Design review of the part built by this model. Coordinates are the model's own, in mm. A direction names the side the tool comes from. Give positions to 0.01 mm unless a question says otherwise; leave off trailing zeros. Loops run counter-clockwise (first coordinate to the right, second up) from the corner with the lowest first, then second, coordinate; pieces in that order, holes last. Notation, with made-up numbers: (-14, 12) - (-1, 12) arc R16 cw to (-1, 35) - close; hole circle Ø2 at (42, -3.75). An arc over 180 degrees is marked (long way). Write each question's results on one line, items separated by ' | '.
```python
from build123d import *

# Parameters (mm, degrees)
DODANIE_WYCI_GNI_CIE1_DEPTH = 900
SKORUPA1_T                  = -10
SZKIC4_R                    = 12
DODANIE_WYCI_GNI_CIE3_DEPTH = 15
SZKIC6_R                    = 12
SZKIC6_R_2                  = 8.15
DODANIE_WYCI_GNI_CIE4_DEPTH = 10
ZAOKR_GLENIE3_R             = 45
SZKIC8_R                    = 20
WYTNIJ_WYCI_GNI_CIE1_DEPTH  = 7.5
SZKIC11_R                   = 20
WYTNIJ_WYCI_GNI_CIE2_DEPTH  = 5
SZKIC12_R                   = 20
WYTNIJ_WYCI_GNI_CIE3_DEPTH  = 5
SZKIC13_R                   = 20
WYTNIJ_WYCI_GNI_CIE4_DEPTH  = 7.5
ZAOKR_GLENIE4_R             = 10
ZAOKR_GLENIE5_R             = 10


with BuildPart() as part:
    # Szkic1 → Dodanie-wyciągnięcie1 (new body)
    with BuildSketch(Plane.XY):
        with BuildLine():
            Line((-469.846310393, -171.010071663), (0, 0))
            Line((0, 0), (0, -500))
            ThreePointArc((0, -500), (-286.788218176, -409.576022144), (-469.846310393, -171.010071663))
        make_face()
    extrude(amount=DODANIE_WYCI_GNI_CIE1_DEPTH)

    # Skorupa1
    skorupa1_openings = [part.faces().sort_by_distance(p)[0] for p in [
        (-179.521279962, -256.382958146, 900),
        (-179.521279962, -256.382958146, 0),
        (-234.923155196, -85.505035831, 450),
        (0, -250, 450),
    ]]
    offset(amount=SKORUPA1_T, openings=skorupa1_openings, kind=Kind.INTERSECTION)

    # Szkic4 → Dodanie-wyciągnięcie3 (add)
    with BuildSketch(Plane(origin=(0, 0, 0), x_dir=(-1, 0, 0), z_dir=(0, 0, -1))):
        with BuildLine():
            Line((0, -20), (0, -490))
            ThreePointArc((0, -490), (281.052453812, -401.384501702), (460.449384185, -167.58987023))
            Line((460.449384185, -167.58987023), (18.793852416, -6.840402867))
            ThreePointArc((18.793852416, -6.840402867), (-11.471528727, 16.383040886), (0, -20))
        make_face()
        Circle(SZKIC4_R, mode=Mode.SUBTRACT)
    dodanie_wyci_gni_cie3 = extrude(amount=-DODANIE_WYCI_GNI_CIE3_DEPTH)

    # Lustro1: Dodanie-wyciągnięcie3 across plane
    add(dodanie_wyci_gni_cie3.mirror(Plane.XY.offset(450)))

    # Szkic6 → Dodanie-wyciągnięcie4 (add)
    with BuildSketch(Plane.XY.offset(440)):
        with BuildLine():
            Line((-18.793852416, -6.840402867), (-460.449384185, -167.58987023))
            ThreePointArc((-460.449384185, -167.58987023), (-281.052453812, -401.384501702), (0, -490))
            Line((0, -490), (0, -20))
            ThreePointArc((0, -20), (11.471528727, 16.383040886), (-18.793852416, -6.840402867))
        make_face()
        with Locations(Location((0, 0, 0), (0, 0, 180))):
            Circle(SZKIC6_R, mode=Mode.SUBTRACT)
        with Locations((-190.094997116, -90.472476083)):
            Circle(SZKIC6_R_2, mode=Mode.SUBTRACT)
        with BuildLine():
            Line((-20, -28.562960135), (-20, -469.574275275))
            ThreePointArc((-20, -469.574275275), (-269.580925085, -385.001460816), (-434.41507852, -179.397713347))
            Line((-434.41507852, -179.397713347), (-208.888849532, -97.312878949))
            ThreePointArc((-208.888849532, -97.312878949), (-183.254594249, -109.266328498), (-171.3011447, -83.632073216))
            Line((-171.3011447, -83.632073216), (-20, -28.562960135))
        make_face(mode=Mode.SUBTRACT)
    dodanie_wyci_gni_cie4 = extrude(amount=-DODANIE_WYCI_GNI_CIE4_DEPTH)

    # Lustro6: Dodanie-wyciągnięcie4 across plane
    add(dodanie_wyci_gni_cie4.mirror(Plane.XY.offset(450)))

    # Zaokrąglenie3
    zaokr_glenie3_edges = [part.edges().sort_by_distance(p)[0] for p in [
        (-434.41507852, -179.397713347, 435),
        (-20, -28.562960135, 435),
        (-20, -469.574275275, 435),
        (-20, -469.574275275, 465),
        (-20, -28.562960135, 465),
        (-434.41507852, -179.397713347, 465),
    ]]
    fillet(zaokr_glenie3_edges, radius=ZAOKR_GLENIE3_R)

    # Szkic8 → Wytnij-wyciągnięcie1 (cut)
    with BuildSketch(Plane(origin=(0, 0, 0), x_dir=(-1, 0, 0), z_dir=(0, 0, -1))):
        Circle(SZKIC8_R)
    extrude(amount=-WYTNIJ_WYCI_GNI_CIE1_DEPTH, mode=Mode.SUBTRACT)

    # Szkic11 → Wytnij-wyciągnięcie2 (cut)
    with BuildSketch(Plane(origin=(0, 0, 430), x_dir=(-1, 0, 0), z_dir=(0, 0, -1))):
        Circle(SZKIC11_R)
    extrude(amount=-WYTNIJ_WYCI_GNI_CIE2_DEPTH, mode=Mode.SUBTRACT)

    # Szkic12 → Wytnij-wyciągnięcie3 (cut)
    with BuildSketch(Plane(origin=(0, 0, 460), x_dir=(-1, 0, 0), z_dir=(0, 0, -1))):
        Circle(SZKIC12_R)
    extrude(amount=-WYTNIJ_WYCI_GNI_CIE3_DEPTH, mode=Mode.SUBTRACT)

    # Szkic13 → Wytnij-wyciągnięcie4 (cut)
    with BuildSketch(Plane(origin=(0, 0, 885), x_dir=(-1, 0, 0), z_dir=(0, 0, -1))):
        Circle(SZKIC13_R)
    extrude(amount=-WYTNIJ_WYCI_GNI_CIE4_DEPTH, mode=Mode.SUBTRACT)

    # Zaokrąglenie4
    zaokr_glenie4_edges = [part.edges().sort_by_distance(p)[0] for p in [
        (-18.793852416, -6.840402867, 437.5),
        (-18.793852416, -6.840402867, 896.25),
        (-18.793852416, -6.840402867, 11.25),
        (-18.793852416, -6.840402867, 467.5),
    ]]
    fillet(zaokr_glenie4_edges, radius=ZAOKR_GLENIE4_R)

    # Zaokrąglenie5
    zaokr_glenie5_edges = [part.edges().sort_by_distance(p)[0] for p in [
        (-208.888849532, -97.312878949, 435),
        (-171.3011447, -83.632073216, 435),
        (-171.3011447, -83.632073216, 465),
        (-208.888849532, -97.312878949, 465),
    ]]
    fillet(zaokr_glenie5_edges, radius=ZAOKR_GLENIE5_R)


solid = part.part
```
Item 1: Clearance check with flat-ended pins moving along their axes: P1, Ø12, axis at x = -106.5, z = 753, coming from the +Y side; P2, Ø5, axis at x = -293.5, z = 207.5, coming from the -Y side; P3, Ø6, axis at x = -145, z = 360, coming from the +Y side. State where each tip first meets the part, or that it passes through.
Output values:
P1: stops at y = -476.91 | P2: stops at y = -406.59 | P3: stops at y = -467.11
Item 2: Wall thickness on probe 1 along Z at (x, y) = (-413.5, -232); probe 2 along Z at (x, y) = (-243, -360); probe 3 along X at (y, z) = (0, 896): over which ranges is each line inside the solid? List them lowest first.
Output values:
probe 1: z = 0 to 15, 430 to 440, 460 to 470, 885 to 900 | probe 2: z = 0 to 15, 885 to 900 | probe 3: x = -20 to -12, 12 to 20
Item 3: Draft analysis for pull direction Z (two halves, no side actions). For faces 1 (the face through (0, -258.9, 885.4)), 2 (the face through (-180, -104, 460)), 3 (the face through (-167, -236, 900)), state which applies: +Z half, -Z half, draft (parallel to the pull), parting line (faces both ways), or undercut.
Output values:
face 1: draft | face 2: undercut | face 3: +Z half
Item 4: We need section C-C on z = 340. Give the boundary of the cut face in (x, y).
Output values:
outline: (-469.85, -171.01) arc R500 ccw to (0, -500) - (0, -490) arc R490 cw to (-460.45, -167.59) - close
Item 5: We need section B-B on x = -56. Give the boundary of the cut face in (y, z).
Output values:
outline: (-496.85, 0) - (-20.38, 0) - (-20.38, 15) - (-486.79, 15) - (-486.79, 430) - (-464.09, 430) - (-464.09, 440) - (-486.79, 440) - (-486.79, 460) - (-464.09, 460) - (-464.09, 470) - (-486.79, 470) - (-486.79, 885) - (-20.38, 885) - (-20.38, 900) - (-496.85, 900) - close; (-48.74, 430) - (-20.38, 430) - (-20.38, 440) - (-48.74, 440) - close; (-48.74, 460) - (-20.38, 460) - (-20.38, 470) - (-48.74, 470) - close
Item 6: We need section A-A on y = -245. Give the boundary of the cut face in (x, z).
Output values:
outline: (-435.86, 0) - (0, 0) - (0, 15) - (-424.35, 15) - (-424.35, 430) - (-401.09, 430) - (-401.09, 440) - (-424.35, 440) - (-424.35, 460) - (-401.09, 460) - (-401.09, 470) - (-424.35, 470) - (-424.35, 885) - (0, 885) - (0, 900) - (-435.86, 900) - close; (-20, 430) - (0, 430) - (0, 440) - (-20, 440) - close; (-20, 460) - (0, 460) - (0, 470) - (-20, 470) - close
Item 7: Tool access review of faces 4 (the face through (-277.61, -403.773, 219.595)), 5 (the face through (-122.536, -65.883, 464.93)), 6 (the face through (-179, -250, 0)): name each direction out of +Z, -Z, +X, -X, +Y, -Y from which nothing blocks a thin tool from reaching the whole face with its end or side.
Output values:
face 4: +X, +Y | face 5: none | face 6: -Z, +X, -X, +Y, -Y
